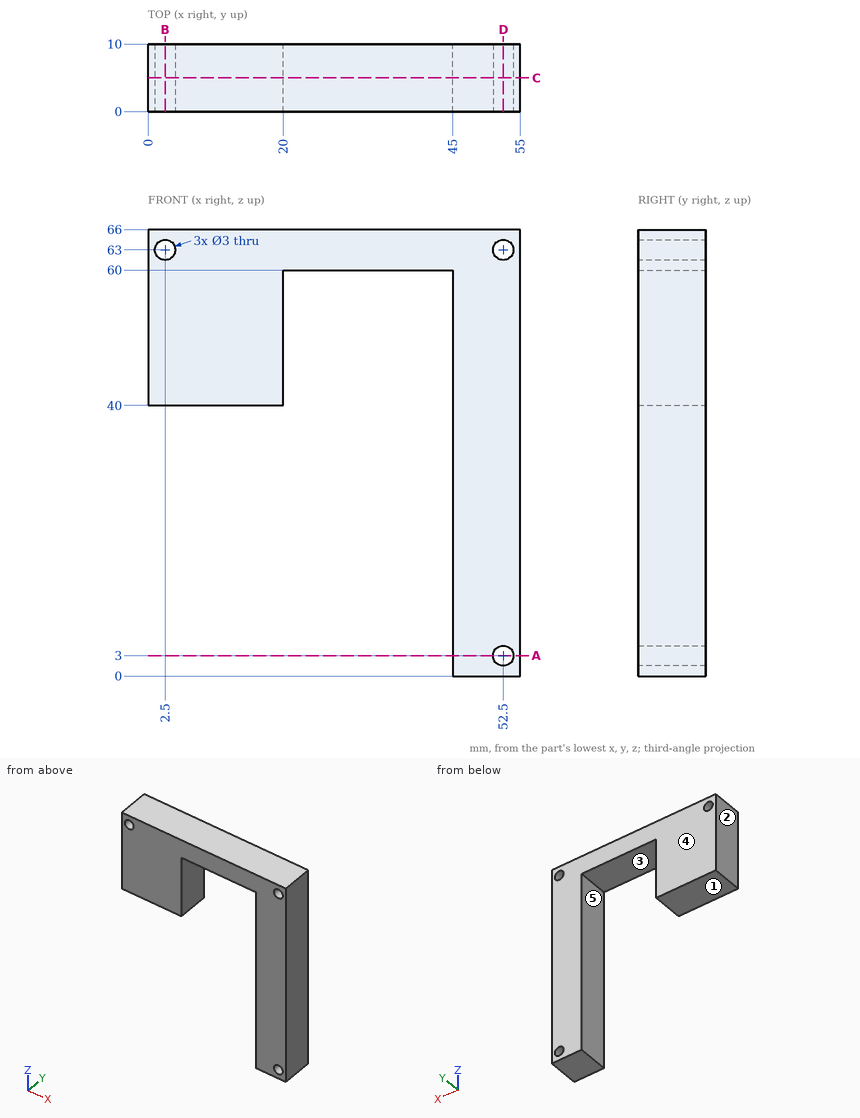
Design review of the part shown in the three views and the two pictorial views. Dimensions are in mm from the part's minimum x, y and z. A direction names the side the tool comes from. Coordinates: 2 decimals unless noted, no trailing zeros. Order: outer loops, then holes, each group sorted by start corner. A loop starts at its lowest first (then second) coordinate and runs counter-clockwise, first axis right, second up. Notation, with made-up numbers: (16, 2) - (61, 2) arc R30 ccw to (61, 32) - close; hole circle Ø10 at (-19.75, 69). An arc over 180 degrees is marked (long way). Answer as CSV lines item,"result". Start each with the question number.
1) Add section A-A (z = 3). State the section outline as (x, y) points, then the cut area to 3 significant figures.
2) Add section B-B (x = 2.5). State the section outline as (y, z) points.
3) Add section C-C (y = 5). State the section outline as (x, z) points, then the cut area to 3 significant figures.
4) Draft analysis for pull direction X (two halves, no side actions). For the marked faces 1, 2 and 3, state which applies: +X half, -X half, draft (parallel to the pull), parting line (faces both ways), or undercut.
5) Insertion check: P1, Ø1, axis at y = 8.5, z = 13.5, coming from the -X side; P2, Ø5, axis at x = 11, y = 3, coming from the -Z side. Each pin has a flat end and moves straight along its axis. Give the tip position at first contact, or say it passes through.
6) Machinability: for the marked faces 4 and 5, which of the approach directions +Z, -Z, +X, -X, +Y, -Y give a long, thin tool a straight path to every point of the face, cutting with its end or side? Answer none if there is none.
7) Add section D-D (x = 52.5). State the section outline as (y, z) points, then the cut area to 3 significant figures.
8) To check wall thickness, follow line 1 along X through (y, z) = (6, 63); line 2 along X through (y, z) = (5.75, 3); line 3 along Z through (x, y) = (13, 0.5). State the ranges of each line that lie inside material, in increasing order. Write a range as [from, to].
Result:
1,outline,"(45, 0) - (51, 0) - (51, 10) - (45, 10) - close; (54, 0) - (55, 0) - (55, 10) - (54, 10) - close"
1,area,"70.0 mm^2"
2,outline,"(0, 40) - (10, 40) - (10, 61.5) - (0, 61.5) - close; (0, 64.5) - (10, 64.5) - (10, 66) - (0, 66) - close"
3,outline,"(0, 40) - (20, 40) - (20, 60) - (45, 60) - (45, 0) - (55, 0) - (55, 66) - (0, 66) - close; hole circle Ø3 at (2.5, 63); hole circle Ø3 at (52.5, 3); hole circle Ø3 at (52.5, 63)"
3,area,"1,310 mm^2"
4,face 1,"draft"
4,face 2,"-X half"
4,face 3,"undercut"
5,P1,"x = 45"
5,P2,"z = 40"
6,face 4,"+Z, -Z, +X, -X, +Y"
6,face 5,"-Z, +Y, -Y"
7,outline,"(0, 0) - (10, 0) - (10, 1.5) - (0, 1.5) - close; (0, 4.5) - (10, 4.5) - (10, 61.5) - (0, 61.5) - close; (0, 64.5) - (10, 64.5) - (10, 66) - (0, 66) - close"
7,area,"600 mm^2"
8,line 1,"[0, 1], [4, 51], [54, 55]"
8,line 2,"[45, 51], [54, 55]"
8,line 3,"[40, 66]"
